Job drawing, mm, ordinate dimensions from the low corner. One solid piece. A direction names the side the tool comes from. Round coordinates to 2 decimals unless told otherwise and drop trailing zeros. Order: outer loops, then holes, each group sorted by start corner. A loop starts at its lowest first (then second) coordinate and runs counter-clockwise, first axis right, second up. Notation, with made-up numbers: (86.5, 67) -> (107.5, 67) arc R21 cw to (107.5, 71) -> close; hole circle Ø11 at (-11, -18.75). An arc over 180 degrees is marked (long way). Return JSON: item names as keys, results as strings. Group by question number.
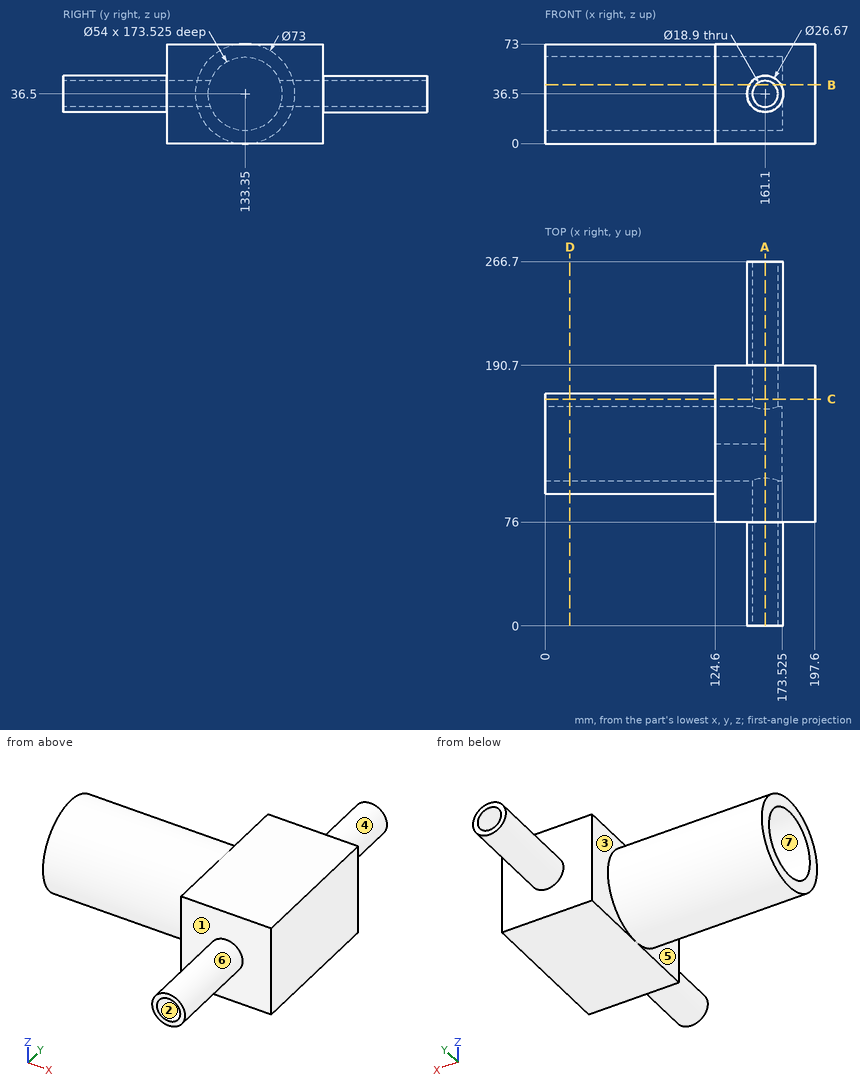
(1) Mould opens along X. For the marked faces 1, 2 and 3 say: pulls with the +X half, pulls with the -X half, needs draft (parallel to the pull), parting line crosses it, or undercut.
(2) Saw through at A-A, the plane x = 161.1. List the corners of the cut face in (y, z) (3 decimals), and give its area (3 significant figures).
(3) Saw through at C-C, the plane y = 166. List the corners of the cut face in (x, z).
(4) Pin check, flat tips, straight feed: P1, Ø3, axis at x = 48.5, z = 49.5, coming from the -Y side; P2, Ø8, axis at y = 75, z = 60.5, coming from the -X side; P3, Ø6, axis at x = 97, z = 18, coming from the +Y side. Stop position of each tip, or through.
(5) Tool access for the marked faces 4, 5, 6 and 7: list every direction of +Z, -Z, +X, -X, +Y, -Y with a clear straight run to the whole face (end or side of a thin tool).
(6) Probe L1, parallel to Y at x = 43.5, z = 36.5; L2, parallel to Z at x = 161, y = 35; L3, parallel to X at y = 25, z = 36. List the from-to ranges inside material, lowest first. Write a range as [from, to].
(7) Saw through at B-B, the plane z = 43. List the corners of the cut face in (x, y) (3 decimals).
(8) Saw through at D-D, the plane x = 18. List the corners of the cut face in (y, z), and give its area (3 significant figures).
Results are:
{
 "1": {"face 1": "needs draft", "face 2": "undercut", "face 3": "pulls with the -X half"},
 "2": {"outline": "(0, 23.165) -> (76, 23.165) -> (76, 0) -> (190.7, 0) -> (190.7, 23.165) -> (266.7, 23.165) -> (266.7, 27.05) -> (158.642, 27.05) arc R27 cw to (108.058, 27.05) -> (0, 27.05) -> close; (0, 45.95) -> (108.058, 45.95) arc R27 cw to (158.642, 45.95) -> (266.7, 45.95) -> (266.7, 49.835) -> (190.7, 49.835) -> (190.7, 73) -> (76, 73) -> (76, 49.835) -> (0, 49.835) -> close", "area": "6,100 mm^2"},
 "3": {"outline": "(0, 20.18) -> (124.6, 20.18) -> (124.6, 0) -> (197.6, 0) -> (197.6, 73) -> (124.6, 73) -> (124.6, 52.82) -> (0, 52.82) -> close; hole circle Ø18.9 at (161.1, 36.5)"},
 "4": {"P1": "stops at y = 98.71", "P2": "stops at x = 124.6", "P3": "stops at y = 166.4"},
 "5": {"face 4": "+Y", "face 5": "-X, -Y", "face 6": "-Y", "face 7": "-X"},
 "6": {"L1": "y = [96.85, 106.35], [160.35, 169.85]", "L2": "z = [23.17, 27.05], [45.95, 49.83]", "L3": "x = [147.77, 151.66], [170.54, 174.43]"},
 "7": {"outline": "(0, 97.433) -> (124.6, 97.433) -> (124.6, 76) -> (149.456, 76) -> (149.456, 0) -> (154.241, 0) -> (154.241, 107.144) -> (0, 107.144) -> close; (0, 159.556) -> (154.241, 159.556) -> (154.241, 266.7) -> (149.456, 266.7) -> (149.456, 190.7) -> (124.6, 190.7) -> (124.6, 169.267) -> (0, 169.267) -> close; (167.959, 0) -> (172.744, 0) -> (172.744, 76) -> (197.6, 76) -> (197.6, 190.7) -> (172.744, 190.7) -> (172.744, 266.7) -> (167.959, 266.7) -> (167.959, 159.556) -> (173.525, 159.556) -> (173.525, 107.144) -> (167.959, 107.144) -> close"},
 "8": {"outline": "circle Ø73 at (133.35, 36.5); hole circle Ø54 at (133.35, 36.5)", "area": "1,900 mm^2"}
}
